Geometry check sheet. Reference: the model listing, model coordinates, mm. A direction names the side the tool comes from. Round coordinates to 2 decimals unless told otherwise and drop trailing zeros. Loops run counter-clockwise (first coordinate to the right, second up) from the corner with the lowest first, then second, coordinate; pieces in that order, holes last. Notation, with made-up numbers: (70, -32) -> (119, -32) arc R23 cw to (119, -24) -> close; hole circle Ø5 at (7, 76). An arc over 180 degrees is marked (long way). Use a Markdown table: item, result. Add a question column.
Q1. Sectioned sample at A-A, the plane y = -9. Enter the section's corners in (x, z).
Q2. Gauge pin test, flat ends, axial feed: P1, Ø10, axis at x = 36, y = -23.5, coming from the +Z side; P2, Ø8, axis at x = 69.5, y = 1.5, coming from the +Z side; P3, Ø6, axis at x = 44, z = 12, coming from the -Y side. Record the tip position at first contact, or that the pin passes through.
Q3. Sectioned sample at C-C, the plane x = -34.5. Enter the section's corners in (y, z).
Q4. Material ranges on L1, parallel to Y at x = 56, z = 4.5; L2, parallel to X at y = -20, z = 10.75; L3, parallel to Z at x = 43, y = -8.5, recorded low to high.
Q5. Sectioned sample at B-B, the plane x = 51. Enter the section's corners in (y, z).
Q6. Set-up check for faces 1 (the face through (99, -5, 10)), 2 (the face through (70, -5, 10)), 3 (the face through (-56.494, -6, 2)): record each of +Z, -Z, +X, -X, +Y, -Y from which the full face is reachable in a straight line by a thin tool's end or side.
```python
from build123d import *

# Parameters (mm, degrees)
SKETCH1_W                = 199.90213939
SKETCH1_H                = 34.765589459
BOSS_EXTRUDE1_DEPTH      = 10
BOSS_EXTRUDE2_DEPTH      = 5
BOSS_EXTRUDE2_DEPTH_BACK = 40
SKETCH2_R                = 9.143615086
DOME1_FACE_RADIUS        = 9.143615086
DOME1_HEIGHT             = 10
DOME2_FACE_RADIUS        = 9.143615086
DOME2_HEIGHT             = 10
CUT_EXTRUDE1_DEPTH       = 54


with BuildPart() as part:
    # Sketch1 → Boss-Extrude1 (new body)
    with BuildSketch(Plane.XY):
        with Locations((43.456986824, -5.3114095)):
            Rectangle(SKETCH1_W, SKETCH1_H)
    extrude(amount=BOSS_EXTRUDE1_DEPTH)

    # Sketch2 → Boss-Extrude2 (add, two sides: drawn at the far end of the back side and taken through both)
    with BuildSketch(Plane(origin=(0, 12.071385229, 0), x_dir=(1, 0, 0), z_dir=(0, 1, 0)).offset(-BOSS_EXTRUDE2_DEPTH_BACK)):
        with Locations(Location((86.99978083, -10, 0), (0, 0, 270))):
            Circle(SKETCH2_R)
    extrude(amount=BOSS_EXTRUDE2_DEPTH + BOSS_EXTRUDE2_DEPTH_BACK)

    # Dome1: an elliptical dome of height H over a round flat face of radius A is half a spheroid: the quarter ellipse of half axes A and H revolved about the face's axis
    with BuildSketch(Plane((86.99978083, 17.071385229, 10), x_dir=(0, 0, -1), z_dir=(1, 0, 0)), mode=Mode.PRIVATE) as dome1_quarter:
        Ellipse(DOME1_FACE_RADIUS, DOME1_HEIGHT)
        Rectangle(DOME1_FACE_RADIUS, DOME1_HEIGHT, align=(Align.MIN, Align.MIN), mode=Mode.INTERSECT)
    revolve(dome1_quarter.sketch, axis=Axis((86.99978083, 17.071385229, 10), (0, 1, 0)))

    # Dome2: an elliptical dome of height H over a round flat face of radius A is half a spheroid: the quarter ellipse of half axes A and H revolved about the face's axis
    with BuildSketch(Plane((86.99978083, -27.928614771, 10), x_dir=(0, 0, 1), z_dir=(1, 0, 0)), mode=Mode.PRIVATE) as dome2_quarter:
        Ellipse(DOME2_FACE_RADIUS, DOME2_HEIGHT)
        Rectangle(DOME2_FACE_RADIUS, DOME2_HEIGHT, align=(Align.MIN, Align.MIN), mode=Mode.INTERSECT)
    revolve(dome2_quarter.sketch, axis=Axis((86.99978083, -27.928614771, 10), (0, -1, 0)))

    # Sketch3 → Cut-Extrude1 (cut)
    with BuildSketch(Plane(origin=(0, 12.071385229, 0), x_dir=(1, 0, 0), z_dir=(0, 1, 0))):
        Polygon((-56.494082871, -5), (61.988701151, -10), (-56.494082871, -10), align=None)
        Polygon((143.408056519, -5), (102.312904095, -10), (143.408056519, -10), align=None)
    extrude(amount=-CUT_EXTRUDE1_DEPTH, mode=Mode.SUBTRACT)


solid = part.part
```
Values:
| question | item | result |
|---|---|---|
| 1 | outline | (-56.49, 0) -> (143.41, 0) -> (143.41, 5) -> (102.31, 10) -> (96.14, 10) arc R9.14 ccw to (77.86, 10) -> (61.99, 10) -> (-56.49, 5) -> close |
| 2 | P1 | z = 9.11 |
| 2 | P2 | z = 10 |
| 2 | P3 | y = -22.69 |
| 3 | outline | (-22.69, 0) -> (12.07, 0) -> (12.07, 5.93) -> (-22.69, 5.93) -> close |
| 4 | L1 | -22.69 to 12.07 |
| 4 | L2 | 77.89 to 96.11 |
| 4 | L3 | 0 to 9.2 |
| 5 | outline | (-22.69, 0) -> (12.07, 0) -> (12.07, 9.54) -> (-22.69, 9.54) -> close |
| 6 | face 1 | +Z, +X, +Y, -Y |
| 6 | face 2 | +Z, -X, +Y, -Y |
| 6 | face 3 | +Z, -Z, -X, +Y, -Y |
